Input: part model. Units: mm. Frame: model coordinates. Round coordinates to 2 decimals unless told otherwise and drop trailing zeros. Loops run counter-clockwise (first coordinate to the right, second up) from the corner with the lowest first, then second, coordinate; pieces in that order, holes last. Notation, with made-up numbers: (45.5, 24.25) -> (79.5, 24.25) arc R25 ccw to (79.5, 38.25) -> close; hole circle Ø2 at (43, -3). An arc over 180 degrees is marked (long way). Answer as a JSON object with one key per item and string values. Group by question number.
Item 1: Pin query (flat end, axial travel): pin 1 (0.8 mm diameter, centred on x = -9.5, y = -42.5, fed in from -Z); pin 2 (3 mm diameter, centred on x = 0, z = 0, fed in from +Y) (3 decimals); pin 3 (2.5 mm diameter, centred on x = 0, y = -50, fed in from -Z); pin 4 (10 mm diameter, centred on y = -37.5, z = -2, fed in from -X). Return the tip coordinate at first contact, or that it passes through.
Item 2: Section query B-B on z = 0. Return loops of the section in (x, y), and give its area (3 significant figures).
Item 3: Material intervals for line 1 (X direction, y = -8, z = 7.5); line 2 (X direction, y = -10.5, z = -8.5); line 3 (X direction, y = -115, z = -4.75), sorted ascending. Write a range as [from, to].
Item 4: Section query A-A on x = 0. Return loops of the section in (y, z).
from build123d import *

# Parameters (mm, degrees)
SALIENTE_EXTRUIR1_START = -141.5
SALIENTE_EXTRUIR1_DEPTH = 283
CROQUIS2_R              = 2.5
CORTAR_EXTRUIR1_DEPTH   = 284.356342905


# Read off the part's stored shape, not the designer's step: Saliente-Extruir1
with BuildPart() as part:
    # Saliente-Extruir1 outline → Saliente-Extruir1 (new body)
    with BuildSketch(Plane(origin=(0, 0, 0), x_dir=(1, 0, 0), z_dir=(0, 1, 0)).offset(SALIENTE_EXTRUIR1_START)):
        with BuildLine():
            ThreePointArc((8.636410676, -9.909743891), (9.614405544, -9.524074441), (10, -8.546050003))
            Line((10, -8.546050003), (10, -3.656511811))
            Line((10, -3.656511811), (9.639909344, -3.656484199))
            Line((9.639909344, -3.656484199), (9.639947683, -3.156497817))
            Line((9.639947683, -3.156497817), (8.092374533, -3.156379149))
            Line((8.092374533, -3.156379149), (8.092195869, -5.486379142))
            Line((8.092195869, -5.486379142), (6.812195872, -5.486280992))
            Line((6.812195872, -5.486280992), (3.799920985, -2.474006104))
            Line((3.799920985, -2.474006104), (3.841542046, -2.432385043))
            Line((3.841542046, -2.432385043), (3.841542046, 2.432385043))
            Line((3.841542046, 2.432385043), (3.97749414, 2.474006104))
            Line((3.97749414, 2.474006104), (6.99, 5.486050003))
            Line((6.99, 5.486050003), (8.27, 5.486050003))
            Line((8.27, 5.486050003), (8.27, 3.156050003))
            Line((8.27, 3.156050003), (9.64, 3.156050003))
            Line((9.64, 3.156050003), (9.64, 3.656050003))
            Line((9.64, 3.656050003), (10, 3.656050003))
            Line((10, 3.656050003), (10, 8.546050003))
            ThreePointArc((10, 8.546050003), (9.645746662, 9.491640567), (8.726602194, 9.909743891))
            Line((8.726602194, 9.909743891), (3.746410661, 9.909743891))
            Line((3.746410661, 9.909743891), (3.746383085, 9.550118856))
            Line((3.746383085, 9.550118856), (3.246383087, 9.550157196))
            Line((3.246383087, 9.550157196), (3.246278035, 8.1801572))
            Line((3.246278035, 8.1801572), (5.576278029, 8.179978536))
            Line((5.576278029, 8.179978536), (5.576179878, 6.89997854))
            Line((5.576179878, 6.89997854), (2.563904991, 3.887703652))
            Line((2.563904991, 3.887703652), (2.386331835, 3.887703652))
            Line((2.386331835, 3.887703652), (2.371542046, 3.902385043))
            Line((2.371542046, 3.902385043), (-2.549115201, 3.902385043))
            Line((-2.549115201, 3.902385043), (-2.563904991, 3.887703652))
            Line((-2.563904991, 3.887703652), (-5.576179878, 6.89997854))
            Line((-5.576179878, 6.89997854), (-5.576278029, 8.179978536))
            Line((-5.576278029, 8.179978536), (-3.246278035, 8.1801572))
            Line((-3.246278035, 8.1801572), (-3.246383087, 9.550157196))
            Line((-3.246383087, 9.550157196), (-3.746383085, 9.550118856))
            Line((-3.746383085, 9.550118856), (-3.746410661, 9.909743891))
            Line((-3.746410661, 9.909743891), (-8.636410676, 9.909743891))
            ThreePointArc((-8.636410676, 9.909743891), (-9.581900138, 9.555487091), (-10, 8.636443724))
            Line((-10, 8.636443724), (-10, 3.656050003))
            Line((-10, 3.656050003), (-9.64, 3.656050003))
            Line((-9.64, 3.656050003), (-9.64, 3.156050003))
            Line((-9.64, 3.156050003), (-8.27, 3.156050003))
            Line((-8.27, 3.156050003), (-8.27, 5.486050003))
            Line((-8.27, 5.486050003), (-6.99, 5.486050003))
            Line((-6.99, 5.486050003), (-3.97749414, 2.474006104))
            Line((-3.97749414, 2.474006104), (-4.019115201, 2.432385043))
            Line((-4.019115201, 2.432385043), (-4.019115201, -2.432385043))
            Line((-4.019115201, -2.432385043), (-3.97749414, -2.474006104))
            Line((-3.97749414, -2.474006104), (-6.989769028, -5.486280992))
            Line((-6.989769028, -5.486280992), (-8.269769024, -5.486379142))
            Line((-8.269769024, -5.486379142), (-8.269947688, -3.156379149))
            Line((-8.269947688, -3.156379149), (-9.817520839, -3.156497817))
            Line((-9.817520839, -3.156497817), (-9.8174825, -3.656484199))
            Line((-9.8174825, -3.656484199), (-10.177573156, -3.656511811))
            Line((-10.177573156, -3.656511811), (-10.177573156, -8.546050003))
            ThreePointArc((-10.177573156, -8.546050003), (-9.7919787, -9.524074441), (-8.813983831, -9.909743891))
            Line((-8.813983831, -9.909743891), (-3.923983846, -9.910118855))
            Line((-3.923983846, -9.910118855), (-3.923956241, -9.550118856))
            Line((-3.923956241, -9.550118856), (-3.423956243, -9.550157196))
            Line((-3.423956243, -9.550157196), (-3.423851191, -8.1801572))
            Line((-3.423851191, -8.1801572), (-5.57627803, -8.179992152))
            Line((-5.57627803, -8.179992152), (-5.576179878, -6.89997854))
            Line((-5.576179878, -6.89997854), (-2.563904991, -3.887703652))
            Line((-2.563904991, -3.887703652), (-2.549115201, -3.902385043))
            Line((-2.549115201, -3.902385043), (2.371542046, -3.902385043))
            Line((2.371542046, -3.902385043), (2.386331835, -3.887703652))
            Line((2.386331835, -3.887703652), (5.398606723, -6.89997854))
            Line((5.398606723, -6.89997854), (5.398704874, -8.179992152))
            Line((5.398704874, -8.179992152), (3.246278035, -8.1801572))
            Line((3.246278035, -8.1801572), (3.246383087, -9.550157196))
            Line((3.246383087, -9.550157196), (3.746383085, -9.550118856))
            Line((3.746383085, -9.550118856), (3.74641069, -9.910118855))
            Line((3.74641069, -9.910118855), (8.636410676, -9.909743891))
        make_face()
    extrude(amount=SALIENTE_EXTRUIR1_DEPTH)

    # Croquis2 → Cortar-Extruir1 (cut, through all)
    with BuildSketch(Plane(origin=(0, 141.5, 0), x_dir=(1, 0, 0), z_dir=(0, 1, 0))):
        with Locations(Location((0, 0, 0), (0, 0, 270))):
            Circle(CROQUIS2_R)
    extrude(amount=-CORTAR_EXTRUIR1_DEPTH, mode=Mode.SUBTRACT)


solid = part.part
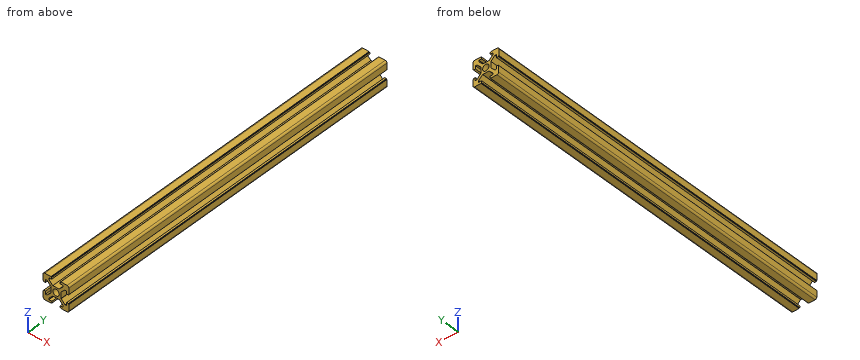
Solved:
{
 "1": {"pin 1": "z = -9.84", "pin 2": "through", "pin 3": "z = -3.9", "pin 4": "x = -10"},
 "2": {"outline": "(-4.02, -141.5) -> (-2.5, -141.5) -> (-2.5, 141.5) -> (-4.02, 141.5) -> close; (2.5, -141.5) -> (3.84, -141.5) -> (3.84, 141.5) -> (2.5, 141.5) -> close", "area": "810 mm²"},
 "3": {"line 1": "[-10.18, -5.58], [5.4, 10]", "line 2": "[-10, -3.25], [3.25, 10]", "line 3": "[-10, -8.27], [-6.25, -3.43], [3.43, 6.25], [8.27, 10]"},
 "4": {"outline": "(-141.5, -3.9) -> (141.5, -3.9) -> (141.5, -2.5) -> (-141.5, -2.5) -> close; (-141.5, 2.5) -> (141.5, 2.5) -> (141.5, 3.9) -> (-141.5, 3.9) -> close"}
}
